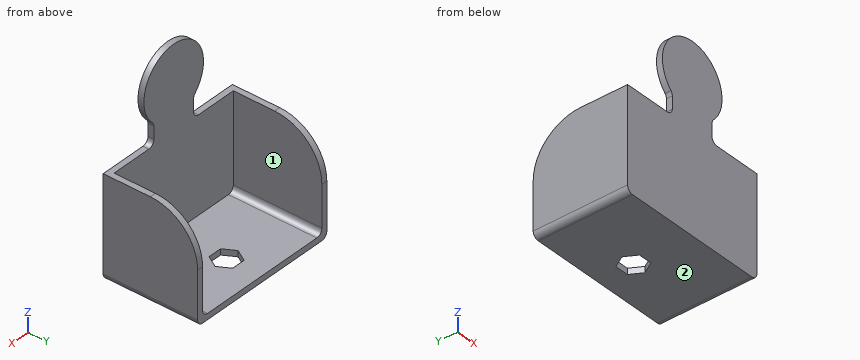
Autodesk Inventor part; units mm, degrees
ref_plane "YZ Plane" through (0, 0, 0) normal (1, 0, 0) x (0, 1, 0)
ref_plane "XZ Plane" through (0, 0, 0) normal (0, 1, 0) x (-1, 0, 0)
ref_plane "XY Plane" through (0, 0, 0) normal (0, 0, 1) x (1, 0, 0)
sketch "Sketch1" plane through (0, 0, 0) normal (0, 1, 0) x (-1, 0, 0)
  line L0 (0, 0) -> (76.2, 0)
  line L1 (76.2, 0) -> (76.2, -50.8)
  line L2 (76.2, -50.8) -> (0, -50.8)
  line L3 (0, -50.8) -> (0, 0)
  line L4 (50.8, 0) -> (25.4, 0)
  line L5 (25.4, 0) -> (25.4, 25.4)
  line L6 (25.4, 25.4) -> (50.8, 25.4)
  line L7 (50.8, 25.4) -> (50.8, 0)
  circle A0 centre (38.1, 25.4) radius 19.05
  point P0 (52.299, 0)
  point P1 (23.901, 0)
  point P2 (50.8, 11.201)
  point P3 (25.4, 11.201)
  dimension "d0" = 76.2
  dimension "d1" = 50.8
  dimension "d2" = 25.4
  dimension "d3" = 25.4
  dimension "d4" = 25.4
  dimension "d5" = 38.1
extrude "Extrusion2" add sketch "Sketch1" along normal blind 3.175
fillet "Fillet2" radius 3.175 4 edges at (-50.8, 1.5875, 11.201) (-50.8, 1.5875, 0) (-25.4, 1.5875, 0) (-25.4, 1.5875, 11.201)
sketch "Sketch2" plane through (0, 0, 0) normal (0, -1, 0) x (1, 0, 0)
  line L0 (0, 0) -> (0, -50.8)
  line L1 (0, 0) -> (3.175, 0)
  line L2 (3.175, 0) -> (3.175, -50.8)
  line L3 (3.175, -50.8) -> (0, -50.8)
  line L4 (0, -50.8) -> (0, 0)
  line L5 (-76.2, -50.8) -> (-76.2, 0)
  line L6 (-76.2, -50.8) -> (-79.375, -50.8)
  line L7 (-79.375, -50.8) -> (-79.375, 0)
  line L8 (-79.375, 0) -> (-76.2, 0)
  line L9 (-76.2, 0) -> (-76.2, -50.8)
  line L10 (3.175, -50.8) -> (-79.375, -50.8)
  line L11 (-79.375, -50.8) -> (-79.375, -53.975)
  line L12 (-79.375, -53.975) -> (3.175, -53.975)
  line L13 (3.175, -53.975) -> (3.175, -50.8)
  dimension "d12" = 3.175
  dimension "d13" = 3.175
  dimension "d14" = 3.175
extrude "Extrusion3" add sketch "Sketch2" against normal blind 50.8
fillet "Fillet3" radius 3.175 4 edges at (3.175, 25.4, -53.975) (-79.375, 25.4, -53.975) (-76.2, 26.9875, -50.8) (0, 26.9875, -50.8)
fillet "Fillet4" radius 25.4 2 edges at (1.5875, 50.8, 0) (-77.7875, 50.8, 0)
ref_plane "Work Plane1" through (-38.1, 0, 0) normal (1, 0, 0) x (0, 0, -1)
sketch "Sketch5" plane through (0, 0, -53.975) normal (0, 0, -1) x (-1, 0, 0)
  line L0 (76.2, 50.8) -> (76.2, 0)
  line L1 (0, 50.8) -> (76.2, 50.8)
  line L2 (0, 0) -> (0, 50.8)
  line L3 (76.2, 0) -> (0, 0)
  line L4 (34.3039, 38.1) -> (41.6363, 38.1)
  line L5 (41.6363, 38.1) -> (45.3025, 31.75)
  line L6 (45.3025, 31.75) -> (41.6363, 25.4)
  line L7 (41.6363, 25.4) -> (34.3039, 25.4)
  line L8 (34.3039, 25.4) -> (30.6378, 31.75)
  line L9 (30.6378, 31.75) -> (34.3039, 38.1)
  line L10 (0, 50.8) -> (76.2, 50.8)
  point P0 (0, 0)
  point P1 (37.9701, 31.75)
  dimension "d27" = 12.7
  dimension "d28" = 12.7
extrude "Extrusion6" cut sketch "Sketch5" against normal blind 25.4 contours L4 L5 L6 L7 L8 L9
properties part number "Prototype Base_3DPrint"
Geometry: final body of the model. Coordinates: model frame, mm. Face numbers are marked on the shaded views. A direction names the side the tool comes from. Give positions to 0.01 mm unless a question says otherwise; leave off trailing zeros. Loops run counter-clockwise (first coordinate to the right, second up) from the corner with the lowest first, then second, coordinate; pieces in that order, holes last. Notation, with made-up numbers: (-9, 71.5) - (50, 71.5) arc R5 cw to (50, 80.5) - close; hole circle Ø3 at (20, 0.25). An arc over 180 degrees is marked (long way). Answer as CSV lines item,"result". Start each with the question number.
(1) Section query C-C (y = 14.5). Output: boundary loops of the cut face in (x, z) (3 decimals).
(2) Ray query, line 1 along X through (y, z) = (9, -16) (3 decimals); line 2 along Z through (x, y) = (-24, 17.5) (3 decimals); line 3 along Y through (x, z) = (-38.5, -11) (3 decimals). Return the intervals inside material, ascending. Write a range as [from, to].
(3) Pin query (flat end, axial travel): P1, Ø2.5, axis at y = 1, z = 6.5, coming from the -X side; P2, Ø2, axis at x = -66.5, z = -19, coming from the +Y side (3 decimals); P3, Ø20.5, axis at x = -67, y = 10, coming from the +Z side. Return the tip coordinate at first contact, or that it passes through.
(4) Section query B-B (y = 30). Output: boundary loops of the cut face in (x, z) (3 decimals), and give its area (3 significant figures).
(5) Reachability of the marked faces 1 and 2 from +Z, -Z, +X, -X, +Y, -Y: full face, straight path, thin tool, end or side. Return the list, or none.
(6) Section query A-A (x = -38.1). Output: boundary loops of the cut face in (y, z) (3 decimals).
(7) Section query D-D (z = 25.4). Output: boundary loops of the cut face in (x, y) (3 decimals), and give its area (3 significant figures).
Worked answers:
1,outline,"(-79.375, -50.8) arc R3.175 ccw to (-76.2, -53.975) - (0, -53.975) arc R3.175 ccw to (3.175, -50.8) - (3.175, 0) - (0, 0) - (0, -47.625) arc R3.175 cw to (-3.175, -50.8) - (-73.025, -50.8) arc R3.175 cw to (-76.2, -47.625) - (-76.2, 0) - (-79.375, 0) - close"
2,line 1,"x = [-79.375, -76.2], [0, 3.175]"
2,line 2,"z = [-53.975, -50.8]"
2,line 3,"y = [0, 3.175]"
3,P1,"stops at x = -50.8"
3,P2,"stops at y = 3.175"
3,P3,"stops at z = 0"
4,outline,"(-79.375, -50.8) arc R3.175 ccw to (-76.2, -53.975) - (-44.292, -53.975) - (-44.292, -50.8) - (-73.025, -50.8) arc R3.175 cw to (-76.2, -47.625) - (-76.2, -0.42) - (-79.375, -0.42) - close; (-31.648, -53.975) - (0, -53.975) arc R3.175 ccw to (3.175, -50.8) - (3.175, -0.42) - (0, -0.42) - (0, -47.625) arc R3.175 cw to (-3.175, -50.8) - (-31.648, -50.8) - close"
4,area,"542 mm^2"
5,face 1,"+Z, +Y"
5,face 2,"-Z, +X, -X, +Y, -Y"
6,outline,"(0, -53.975) - (25.4, -53.975) - (25.4, -50.8) - (3.175, -50.8) - (3.175, 44.45) - (0, 44.45) - close; (38.1, -53.975) - (50.8, -53.975) - (50.8, -50.8) - (38.1, -50.8) - close"
7,outline,"(-57.15, 0) - (-19.05, 0) - (-19.05, 3.175) - (-57.15, 3.175) - close"
7,area,"121 mm^2"
